Autodesk Inventor part; units mm, degrees
ref_plane "YZ Plane" through (0, 0, 0) normal (1, 0, 0) x (0, 1, 0)
ref_plane "XZ Plane" through (0, 0, 0) normal (0, 1, 0) x (-1, 0, 0)
ref_plane "XY Plane" through (0, 0, 0) normal (0, 0, 1) x (1, 0, 0)
ref_plane "Work Plane2" through (35.545, -31.609, 1.6) normal (0, 0, 1) x (1, 0, 0)
ref_plane "Work Plane1" through (35.545, -31.609, 1.6) normal (0, 0, 1) x (1, 0, 0)
sketch "Sketch1" plane through (35.545, -31.609, 1.6) normal (0, 0, 1) x (1, 0, 0)
  line L0 (0, 0) -> (336, 0)
  line L1 (-2, -129) -> (-2, -2)
  line L2 (-1.6825, -0.9187) -> (-1.5115, -0.6903)
  arc A0 (0, 0) -> (-2, -2) centre (0, -2) ccw
  line L3 (338, -2) -> (338, -129)
  line L4 (337.5115, -0.6903) -> (337.6825, -0.9187)
  arc A1 (338, -2) -> (336, 0) centre (336, -2) ccw
  line L5 (336, -131) -> (0, -131)
  line L6 (337.6825, -130.0813) -> (337.5115, -130.3097)
  arc A2 (336, -131) -> (338, -129) centre (336, -129) ccw
  arc A3 (-2, -129) -> (0, -131) centre (0, -129) ccw
  circle A4 centre (1.98, -128.63) radius 1.1
  circle A5 centre (1.98, -128.63) radius 1.1
  circle A6 centre (68.313, -128.63) radius 1.1
  circle A7 centre (134.646, -128.63) radius 1.1
  circle A8 centre (134.646, -128.63) radius 1.1
  circle A9 centre (68.313, -128.63) radius 1.1
  circle A10 centre (200.979, -128.63) radius 1.1
  circle A11 centre (267.312, -128.63) radius 1.1
  circle A12 centre (333.645, -128.63) radius 1.1
  circle A13 centre (333.645, -128.63) radius 1.1
  circle A14 centre (267.312, -128.63) radius 1.1
  circle A15 centre (200.979, -128.63) radius 1.1
  circle A16 centre (333.638, -2.355) radius 1.1
  circle A17 centre (1.973, -2.355) radius 1.1
  circle A18 centre (68.306, -2.355) radius 1.1
  circle A19 centre (134.639, -2.355) radius 1.1
  circle A20 centre (200.972, -2.355) radius 1.1
  circle A21 centre (267.305, -2.355) radius 1.1
  circle A22 centre (333.645, -2.355) radius 1.093
  circle A23 centre (267.305, -2.355) radius 1.1
  circle A24 centre (200.972, -2.355) radius 1.1
  circle A25 centre (134.639, -2.355) radius 1.1
  circle A26 centre (68.306, -2.355) radius 1.1
  circle A27 centre (1.973, -2.355) radius 1.1
  line L7 (3, -4.2357) -> (125.2758, -4.2357) construction
  line L8 (4, -5) -> (332, -5)
  line L9 (333, -6) -> (333, -125)
  line L10 (332, -126) -> (4, -126)
  line L11 (3, -125) -> (3, -6)
  arc A28 (4, -5) -> (3, -6) centre (4, -6) ccw
  arc A29 (333, -6) -> (332, -5) centre (332, -6) ccw
  arc A30 (332, -126) -> (333, -125) centre (332, -125) ccw
  arc A31 (3, -125) -> (4, -126) centre (4, -125) ccw
  line L12 (162.5077, 0) -> (162.5077, -5)
  line L13 (173.4174, -5) -> (173.4174, 0)
  circle A32 centre (320.737, -95.692) radius 0.175
  line L14 (333, -88.192) -> (338, -88.192)
  line L15 (333, -102.192) -> (338, -102.192)
  line L16 (257.6125, -126) -> (315.0362, -126)
  line L17 (315.0362, -126) -> (315.0362, -126.7604)
  line L18 (315.0362, -126.7604) -> (257.6125, -126.7604)
  line L19 (257.6125, -126.7604) -> (257.6125, -126)
  point P0 (-35.545, 31.609)
  point P1 (-1.5115, -130.3097)
  point P2 (335.5, -88.192)
  point P3 (0, -131)
  point P4 (337.6825, -130.0813)
  point P5 (-1.6825, -0.9187)
  point P6 (337.6825, -0.9187)
  dimension "d2" = 5
  dimension "d3" = 5
  dimension "d4" = 5
  dimension "d5" = 5
  dimension "d6" = 1
  dimension "d7" = 1
  dimension "d8" = 1
  dimension "d9" = 1
extrude "Extrusion3" add sketch "Sketch1" along normal blind 4.5 contours L0 L12 L8 A28 L11 A31 L10 L19 L18 L17 A30 L9 L15 L3 A2 L6 L5 A3 L1 A0 L2
properties part number "open_liner_L"
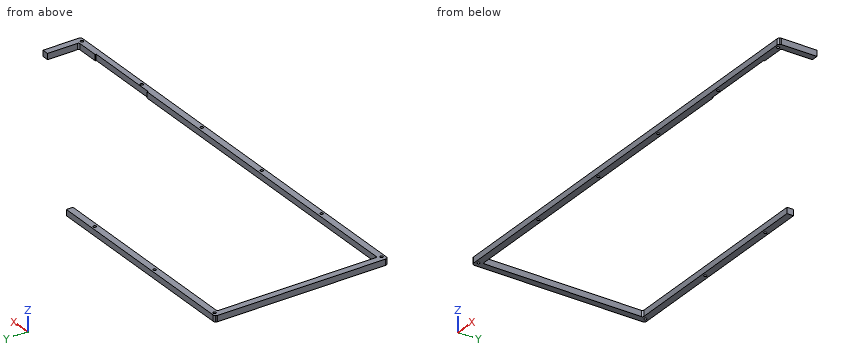
Geometry: final body of the model. Coordinates: model frame, mm. Coordinates: 2 decimals unless noted, no trailing zeros. Write each loop counter-clockwise with the first axis right and the second up, starting at its lowest first coordinate (ties: lowest second). Pieces come first, ordered by that corner, then holes. Notation, with made-up numbers: (-7.75, 21.25) - (37.25, 21.25) arc R30 ccw to (37.25, 51.25) - close; hole circle Ø4 at (58.5, 78). An arc over 180 degrees is marked (long way). Return JSON: item names as keys, results as strings.
Item 1: Section query D-D (y = -113). Output: boundary loops of the cut face in (x, z) (3 decimals), and give its area (3 significant figures).
Completed:
{"outline": "(33.545, 1.6) - (38.545, 1.6) - (38.545, 6.1) - (33.545, 6.1) - close", "area": "22.5 mm2"}
Item 2: Line query: L1, parallel to Y at x = 105, z = 3.5; L2, parallel to X at y = -139, z = 4.7 (3 decimals); L3, parallel to Y at x = 329.5, z = 3.7. Output: solid intervals per line, ascending.
Completed:
{"L1": "y = -162.61 to -157.61, -36.61 to -31.61", "L2": "x = 33.545 to 38.545, 368.545 to 373.545", "L3": "y = -162.61 to -158.37"}
Item 3: Section query A-A (x = 140). Output: boundary loops of the cut face in (y, z).
Completed:
{"outline": "(-162.61, 1.6) - (-157.61, 1.6) - (-157.61, 6.1) - (-162.61, 6.1) - close; (-36.61, 1.6) - (-31.61, 1.6) - (-31.61, 6.1) - (-36.61, 6.1) - close"}
Item 4: Section query C-C (x = 276.5). Output: boundary loops of the cut face in (y, z), and give its area (3 significant figures).
Completed:
{"outline": "(-162.61, 1.6) - (-157.61, 1.6) - (-157.61, 6.1) - (-162.61, 6.1) - close", "area": "22.5 mm2"}
Item 5: Section query B-B (z = 4.8). Count the separate pieces of the cut face and the enclosed holes in it, and give its area (3 significant figures).
Completed:
{"separate pieces": "1", "enclosed holes": "9", "area": "3,170 mm2"}
